Here's how the part is built. I have some questions about the finished solid (model axes, mm). Face numbers are marked on the shaded views. A direction names the side the tool comes from. Coordinates: 2 decimals unless noted, no trailing zeros. Loops run counter-clockwise (first coordinate to the right, second up) from the corner with the lowest first, then second, coordinate; pieces in that order, holes last. Notation, with made-up numbers: (-26, 74.5) -> (23, 74.5) arc R21 cw to (23, 83.5) -> close; hole circle Ø4 at (31, -31). An arc over 180 degrees is marked (long way). Answer as a JSON object with one key per item and string values. Group by question number.
Q1. I want a section at A-A on x = 8. Write out the boundary of the cut face in (y, z).
Q2. I'm going to push flat-ended pins straight in: pin 1 (1 mm diameter, centred on x = -7.5, z = -0.5, fed in from -Y); pin 2 (0.7 mm diameter, centred on x = 10, z = 0, fed in from -Y). Where does each tip first touch, or does it pass through?
Q3. Thinking about a two-plate mould opening in Z: for the marked faces 3, 4 and 5, which applies, released by +Z, released by -Z, zero draft, split by the parting line, or undercut?
Q4. I want a section at B-B on y = -6.75. Write out the boundary of the cut face in (x, z), then the cut area to 3 significant figures.
Q5. On a 3-axis mill with a long thin cutter (end or side, diameter ignored), from which of +Z, -Z, +X, -X, +Y, -Y can I reach the whole of each face in a straight line? I mean the marked faces 1 and 2. Say none if no direction works.
Q6. I need wall thicknesses on line 1 (X direction, y = -4.75, z = 9.5); line 2 (Z direction, x = -11, y = -5.25); line 3 (X direction, y = -8.25, z = -8.25). Which ranges of each line are inside material? Lowest first, please.
Q7. I want a section at C-C on y = -2. Write out the boundary of the cut face in (x, z), then the cut area to 3 significant figures.
Q8. I want a section at D-D on x = -12. Write out the boundary of the cut face in (y, z).
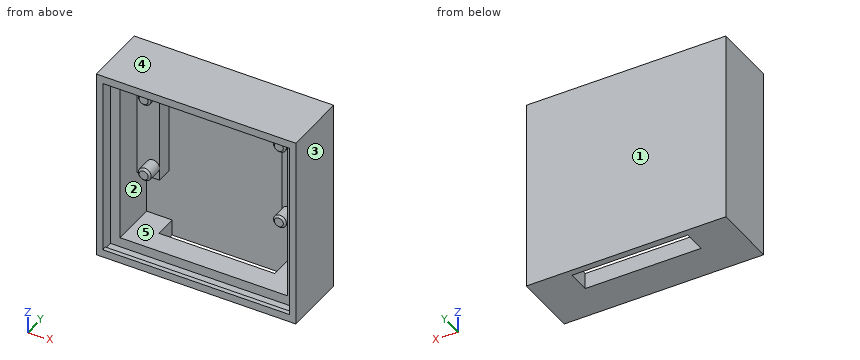
```python
from build123d import *

# Parameters (mm, degrees)
F0_W      = 15.5
F0_H      = 15
F1_DEPTH  = 10
F2_W      = 29
F2_H      = 28
F3_DEPTH  = 2
F4_W      = 26
F4_H      = 25
F5_DEPTH  = 7
F6_W      = 3.5
F6_H      = 17
F7_DEPTH  = 2.5
F8_R      = 1
F9_DEPTH  = 2.5
F10_W     = 18
F10_H     = 3.5
F11_DEPTH = 25
F12_SIZE  = 0.3
F13_W     = 29
F13_H     = 0.7
F14_DEPTH = 0.2
F15_W     = 29
F15_H     = 0.7
F16_DEPTH = 0.2


with BuildPart() as f1:
    # F0 (on Front) → F1 (new body)
    with BuildSketch(Plane.XZ):
        with Locations((-7.75, 10)):
            Rectangle(F0_W, F0_H)
        with Locations((7.75, 10)):
            Rectangle(F0_W, F0_H)
        with Locations((-7.75, -5)):
            Rectangle(F0_W, F0_H)
        with Locations((7.75, -5)):
            Rectangle(F0_W, F0_H)
    extrude(amount=F1_DEPTH)

    # F2 (on face) → F3 (cut)
    with BuildSketch(Plane.XZ.offset(10)):
        with Locations((0, 2.5)):
            Rectangle(F2_W, F2_H)
    extrude(amount=-F3_DEPTH, mode=Mode.SUBTRACT)

    # F4 (on face) → F5 (cut)
    with BuildSketch(Plane.XZ.offset(8)):
        with Locations((0, 2.5)):
            Rectangle(F4_W, F4_H)
    extrude(amount=-F5_DEPTH, mode=Mode.SUBTRACT)

    # F6 (on face) → F7 (join)
    with BuildSketch(Plane.XZ.offset(1)):
        with Locations((-11.25, 6.5)):
            Rectangle(F6_W, F6_H)
        with Locations((11.25, 6.5)):
            Rectangle(F6_W, F6_H)
    extrude(amount=F7_DEPTH)

    # F8 (on face) → F9 (join)
    with BuildSketch(Plane.XZ.offset(3.5)):
        with Locations((-10.5, 12.5)):
            Circle(F8_R)
        with Locations((-10.5, 0)):
            Circle(F8_R)
        with Locations((10.5, 12.5)):
            Circle(F8_R)
        with Locations((10.5, 0)):
            Circle(F8_R)
    extrude(amount=F9_DEPTH)

    # F10 (on face) → F11 (cut)
    with BuildSketch(Plane.XY.offset(-10)):
        with Locations((0, -2.75)):
            Rectangle(F10_W, F10_H)
    extrude(amount=-F11_DEPTH, mode=Mode.SUBTRACT)

    # F12
    f12_edges = [f1.edges().sort_by_distance(p)[0] for p in [
        (-11.5, -6, 12.5),
        (-11.5, -6, 0),
        (9.5, -6, 12.5),
        (9.5, -6, 0),
    ]]
    chamfer(f12_edges, length=F12_SIZE)

    # F13 (on face) → F14 (join)
    with BuildSketch(Plane(origin=(0, 0, 16.5), x_dir=(1, 0, 0), z_dir=(0, 0, -1))):
        with Locations((0, 9.65)):
            Rectangle(F13_W, F13_H)
    extrude(amount=F14_DEPTH)

    # F15 (on face) → F16 (join)
    with BuildSketch(Plane.XY.offset(-11.5)):
        with Locations((0, -9.65)):
            Rectangle(F15_W, F15_H)
    extrude(amount=F16_DEPTH)


solid = f1.part
```
Result set:
{
 "1": {"outline": "(-10, -12.5) -> (-4.5, -12.5) -> (-4.5, -10) -> (-8, -10) -> (-8, -11.5) -> (-9.3, -11.5) -> (-9.3, -11.3) -> (-10, -11.3) -> close; (-10, 16.3) -> (-9.3, 16.3) -> (-9.3, 16.5) -> (-8, 16.5) -> (-8, 15) -> (-1, 15) -> (-1, -12.5) -> (0, -12.5) -> (0, 17.5) -> (-10, 17.5) -> close"},
 "2": {"pin 1": "stops at y = -1", "pin 2": "stops at y = -6"},
 "3": {"face 3": "zero draft", "face 4": "released by +Z", "face 5": "undercut"},
 "4": {"outline": "(-15.5, -12.5) -> (15.5, -12.5) -> (15.5, 17.5) -> (-15.5, 17.5) -> close; hole (-13, -10) -> (13, -10) -> (13, 15) -> (-13, 15) -> close", "area": "280 mm²"},
 "5": {"face 1": "+Z, -Z, +X, -X, +Y", "face 2": "-Y"},
 "6": {"line 1": "x = -15.5 to -13, 13 to 15.5", "line 2": "z = -12.5 to -10, -0.87 to 0.87, 11.63 to 13.37, 15 to 17.5", "line 3": "x = -15.5 to -14.5, 14.5 to 15.5"},
 "7": {"outline": "(-15.5, -12.5) -> (-9, -12.5) -> (-9, -10) -> (-13, -10) -> (-13, -2) -> (-9.5, -2) -> (-9.5, 15) -> (9.5, 15) -> (9.5, -2) -> (13, -2) -> (13, -10) -> (9, -10) -> (9, -12.5) -> (15.5, -12.5) -> (15.5, 17.5) -> (-15.5, 17.5) -> close", "area": "354 mm²"},
 "8": {"outline": "(-10, -12.5) -> (0, -12.5) -> (0, 17.5) -> (-10, 17.5) -> (-10, 16.3) -> (-9.3, 16.3) -> (-9.3, 16.5) -> (-8, 16.5) -> (-8, 15) -> (-3.5, 15) -> (-3.5, -2) -> (-1, -2) -> (-1, -10) -> (-8, -10) -> (-8, -11.5) -> (-9.3, -11.5) -> (-9.3, -11.3) -> (-10, -11.3) -> close"}
}
